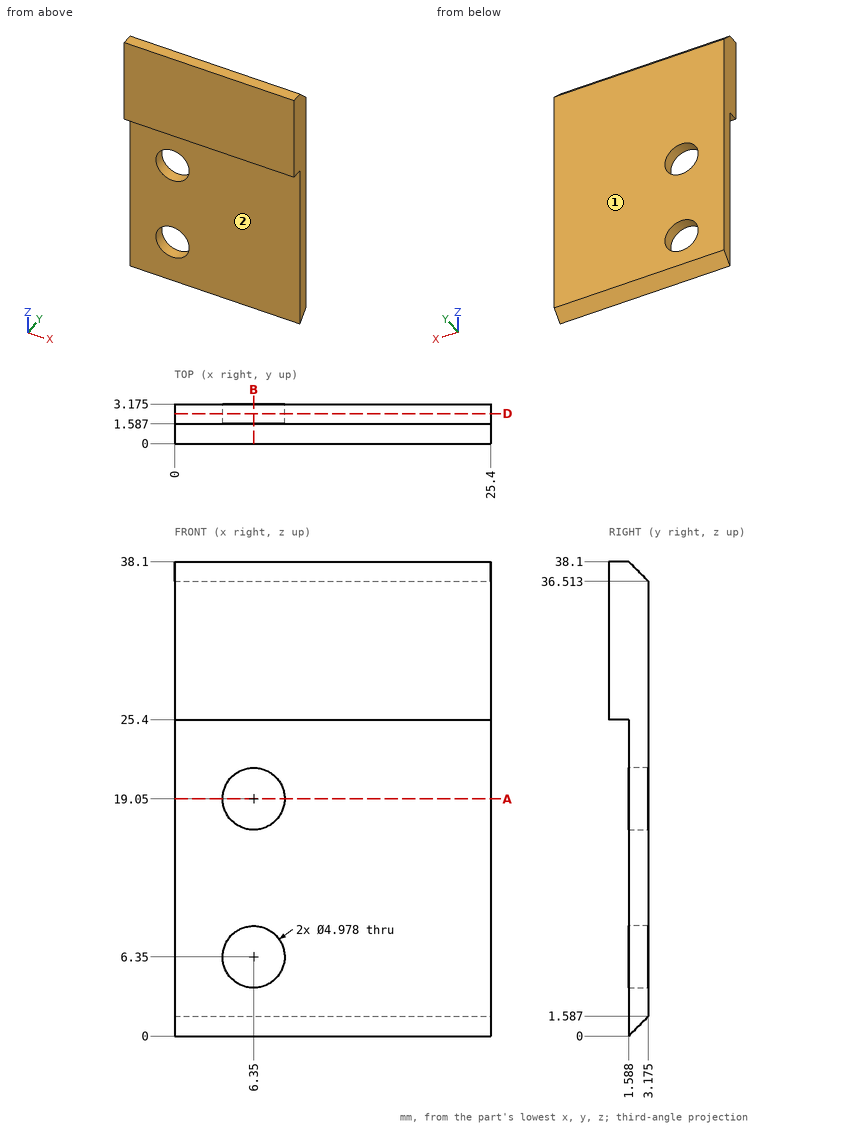
Source: three-view drawing plus pictorial views. Frame: mm from the lowest corner of the part. A direction names the side the tool comes from. Coordinates: 2 decimals unless noted, no trailing zeros. Order: outer loops, then holes, each group sorted by start corner. A loop starts at its lowest first (then second) coordinate and runs counter-clockwise, first axis right, second up.
Item 1: Cut plane B-B (x = 6.35). Count the separate pieces of the cut face and the enclosed holes in it.
Output values:
separate pieces: 3
enclosed holes: 0
Item 2: Cut plane A-A (z = 19.05). Return loops of the section in (x, y) (1 decimal).
Output values:
outline: (0, 1.6) - (3.9, 1.6) - (3.9, 3.2) - (0, 3.2) - close; (8.8, 1.6) - (25.4, 1.6) - (25.4, 3.2) - (8.8, 3.2) - close
Item 3: Material intervals for line 1 (X direction, y = 1.9, z = 6.35); line 2 (Y direction, x = 17, z = 2.5) (1 decimal); line 3 (Z direction, x = 24, y = 0.75), sorted ascending.
Output values:
line 1: x = 0 to 3.86, 8.84 to 25.4
line 2: y = 1.6 to 3.2
line 3: z = 25.4 to 38.1
Item 4: First-contact query: P1, Ø3, axis at x = 6.35, z = 19.05, coming from the -Y side; P2, Ø0.8, axis at x = 16.5, y = 1, coming from the -Z side. Flat tips, straight axial feed; report the tip coordinate or a pass-through.
Output values:
P1: passes through
P2: stops at z = 25.4
Item 5: Set-up query: the marked faces 1 and 2. Return all of +Z, -Z, +X, -X, +Y, -Y with unobstructed straight access to the full face (end or side cutting, diameter ignored); none if empty.
Output values:
face 1: +Z, -Z, +X, -X, +Y
face 2: -Z, +X, -X, -Y
Item 6: Cut plane D-D (y = 2.4). Return loops of the section in (x, z).
Output values:
outline: (0, 0.81) - (25.4, 0.81) - (25.4, 37.29) - (0, 37.29) - close; hole circle Ø4.98 at (6.35, 6.35); hole circle Ø4.98 at (6.35, 19.05)
